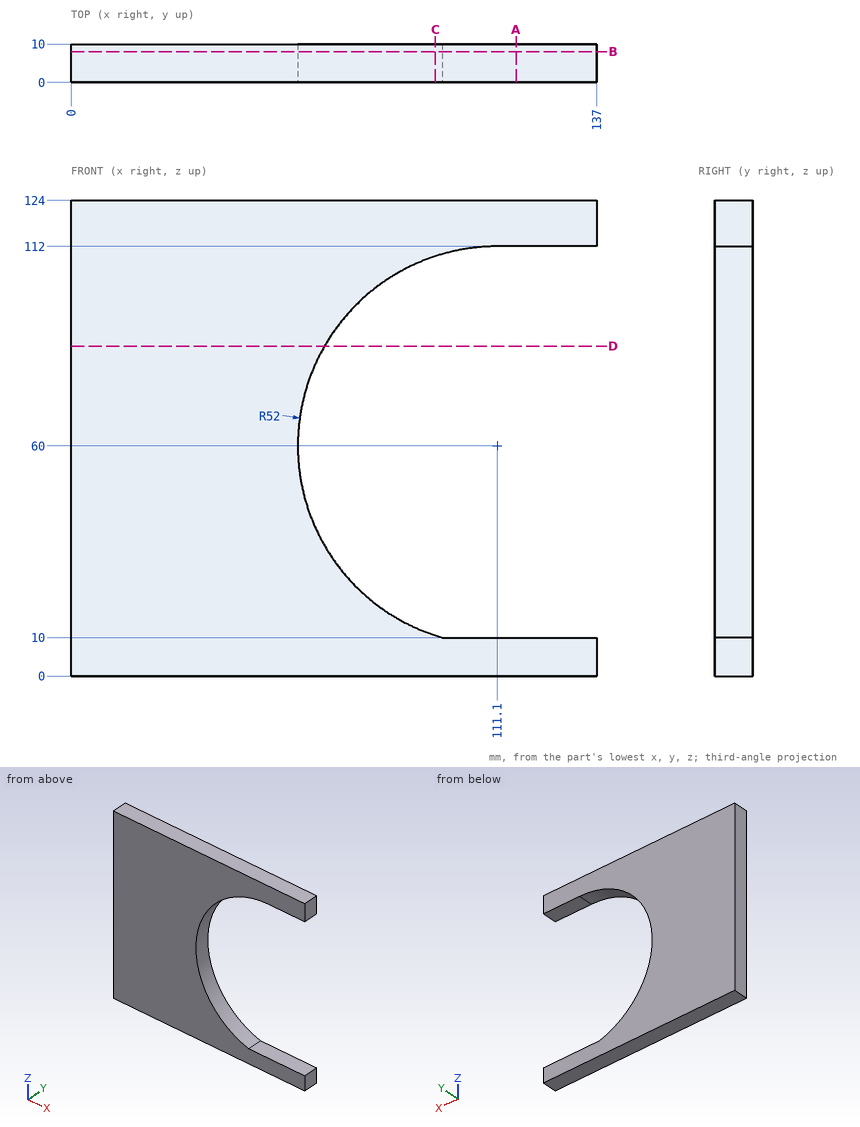
Input: dimensioned drawing with shaded views. Units: mm. Origin: part minimum x, y, z. Give positions to 0.01 mm unless a question says otherwise; leave off trailing zeros. Order: outer loops, then holes, each group sorted by start corner. A loop starts at its lowest first (then second) coordinate and runs counter-clockwise, first axis right, second up. Notation, with made-up numbers: (1.25, 29) -> (15.25, 29) arc R36 ccw to (15.25, 64) -> close; hole circle Ø2 at (0, 82). An arc over 180 degrees is marked (long way). Use a Markdown table: item, result.
1) Section query C-C, the plane x = 95. Return the cut outline in (y, z).
Answer list:
| item | result |
|---|---|
| outline | (0, 0) -> (10, 0) -> (10, 10.56) -> (0, 10.56) -> close; (0, 109.44) -> (10, 109.44) -> (10, 124) -> (0, 124) -> close |
2) Section query A-A, the plane x = 116. Return the cut outline in (y, z), then the cut area to 3 significant figures.
Answer list:
| item | result |
|---|---|
| outline | (0, 0) -> (10, 0) -> (10, 10) -> (0, 10) -> close; (0, 112) -> (10, 112) -> (10, 124) -> (0, 124) -> close |
| area | 220 mm² |
3) Section query B-B, the plane y = 8. Return the cut outline in (x, z).
Answer list:
| item | result |
|---|---|
| outline | (0, 0) -> (137, 0) -> (137, 10) -> (96.82, 10) arc R52 cw to (111.1, 112) -> (137, 112) -> (137, 124) -> (0, 124) -> close |
4) Section query D-D, the plane z = 86. Return the cut outline in (x, y), then the cut area to 3 significant figures.
Answer list:
| item | result |
|---|---|
| outline | (0, 0) -> (66.07, 0) -> (66.07, 10) -> (0, 10) -> close |
| area | 661 mm² |
5) Ray query, line 1 along Z through (x, y) = (117.5, 4.5); line 2 along Z through (x, y) = (65.5, 6); line 3 along X through (y, z) = (9, 39). Return the intervals inside material, ascending. Write a range as [from, to].
Answer list:
| item | result |
|---|---|
| line 1 | [0, 10], [112, 124] |
| line 2 | [0, 35.01], [84.99, 124] |
| line 3 | [0, 63.53] |
